Verification items for the finished model (mm, model axes). A direction names the side the tool comes from. Coordinates: 2 decimals unless noted, no trailing zeros. Loops run counter-clockwise (first coordinate to the right, second up) from the corner with the lowest first, then second, coordinate; pieces in that order, holes last. Notation, with made-up numbers: (32.25, 78.25) - (64.25, 78.25) arc R19 ccw to (64.25, 82.25) - close; hole circle Ø2 at (3.25, 41.5). An arc over 180 degrees is marked (long way). One line per item, written item: value. Start each with the question number.
(1) Draft check along Z on faces 3 (the face through (3.544, -43.056, 40.685)), 4 (the face through (16.244, -69.867, 15.456)), 5 (the face through (3.544, -77.418, 26.011)), 6 (the face through (-2.717, -36, 1)). Enter one of: +Z half, -Z half, draft (parallel to the pull), parting line (faces both ways), or undercut.
(2) Set-up check for faces 1 (the face through (9.983, -22, 1)), 2 (the face through (3.5, -14.1, 0.8)): record each of +Z, -Z, +X, -X, +Y, -Y from which the full face is reachable in a straight line by a thin tool's end or side.
(3) Thickness scan on probe 1 along Z at (x, y) = (7, -58.5); probe 2 along Z at (x, y) = (9.75, -68); probe 3 along Y at (x, z) = (15, 1). Record the ranges inside material, lowest first. Write a range as [from, to].
(4) Section check D-D (z = -56). Record the boundary of the cut face in (x, y), plus the area to 3 significant figures.
(5) Gauge pin test, flat ends, axial feed: P1, Ø10, axis at y = -15.8, z = 24.63, coming from the +X side; P2, Ø14.5, axis at y = -36.76, z = -39.86, coming from the +X side; P3, Ø16.5, axis at y = -91.62, z = 0, coming from the -X side; P4, Ø1, axis at x = 9.5, z = -43.5, coming from the -Y side. Record the tip position at first contact, or that the pin passes through.
(6) Section check B-B (x = 20.75). Record the boundary of the cut face in (y, z) (3 decimals), plus the area to 3 significant figures.
(7) Section check A-A (x = 1.75). Count the separate pieces of the cut face and the enclosed holes in it, plus the area to 3 significant figures.
(8) Section check C-C (z = 49.5). Record the boundary of the cut face in (x, y).
Autodesk Inventor part; units mm, degrees
ref_plane "YZ Plane" through (0, 0, 0) normal (1, 0, 0) x (0, 1, 0)
ref_plane "XZ Plane" through (0, 0, 0) normal (0, 1, 0) x (-1, 0, 0)
ref_plane "XY Plane" through (0, 0, 0) normal (0, 0, 1) x (1, 0, 0)
sketch "Sketch1" plane through (0, 0, 0) normal (0, 0, 1) x (1, 0, 0)
  line L0 (-2.7173, 13.7894) -> (9.9827, 13.7894)
  line L1 (9.9827, 13.7894) -> (9.9827, -24.3106)
  line L2 (9.9827, -40.1856) -> (-2.7173, -40.1856)
  line L3 (-2.7173, -40.1856) -> (-2.7173, 13.7894)
  line L4 (-2.7173, -40.1856) -> (22.6827, -40.1856)
  line L5 (22.6827, -40.1856) -> (22.6827, -24.3106)
  line L6 (22.6827, -24.3106) -> (9.9827, -24.3106)
  line L7 (-2.7173, -24.3106) -> (-2.7173, -40.1856)
  line L8 (-16.1487, -49.7106) -> (31.6829, -49.7106)
  point P0 (0, 0)
  dimension "d0" = 12.7
  dimension "d1" = 53.975
  dimension "d4" = 25.4
  dimension "d5" = 15.875
  dimension "d6" = 9.525
revolve "Revolution1" add sketch "Sketch1" angle 360 about axis through (-16.1487, -49.7106, 0) along (1, 0, 0)
sketch "Sketch3" plane through (22.6827, -49.7106, 0) normal (1, 0, 0) x (0, 0, -1)
  line L0 (0, 11.43) -> (-1.27, 11.43)
  line L1 (0, 11.43) -> (1.27, 11.43)
  line L2 (1.27, 11.43) -> (1.27, 9.44)
  circle A0 centre (0, 0) radius 9.525
  line L3 (-1.27, 11.43) -> (-1.27, 9.44)
  line L4 (1.27, 9.44) -> (-1.27, 9.44)
  point P0 (0, 49.7106)
  dimension "d9" = 1.27
  dimension "d10" = 1.27
extrude "Extrusion1" cut sketch "Sketch3" against normal blind 25.4 contours L1 L2 A0 L3 L0
sketch "Sketch7" plane through (22.6827, -49.7106, 0) normal (1, 0, 0) x (0, 0, -1)
  point P0 (0, 49.7106)
  point P1 (0, 0)
  point P2 (0, 41.91)
  point P3 (-24.6341, 33.9059)
  point P4 (-39.8588, 12.9509)
  point P5 (-39.8588, -12.9509)
  point P6 (-24.6341, -33.9059)
  point P7 (0, -41.91)
  point P8 (24.6341, -33.9059)
  point P9 (39.8588, -12.9509)
  point P10 (39.8588, 12.9509)
  point P11 (24.6341, 33.9059)
  dimension "d29" = 41.91
  dimension "d32" = 360
hole "Hole3" at (22.6827, -49.7106, 0) at (22.6827, -7.8006, 0) at (22.6827, -15.8047, 24.6341) at (22.6827, -36.7597, 39.8588) at (22.6827, -62.6615, 39.8588) at (22.6827, -83.6165, 24.6341) at (22.6827, -91.6206, 0) at (22.6827, -83.6165, -24.6341) at (22.6827, -62.6615, -39.8588) at (22.6827, -36.7597, -39.8588) at (22.6827, -15.8047, -24.6341) direction (-1, 0, 0) diameter 12.7 end through all
properties part number "arthurWeiActivity 5.5a#4.dwg"
Responses:
1. face 3: undercut
1. face 4: parting line
1. face 5: undercut
1. face 6: draft
2. face 1: +X
2. face 2: +X, -X
3. probe 1: z = [-62.89, -44.66], [-35.06, -3.67], [3.67, 35.06], [44.66, 62.89]
3. probe 2: z = [-60.81, -43.3], [-36.42, 36.42], [43.3, 60.81]
3. probe 3: y = [-75.09, -59.18], [-38.28, -24.33]
4. outline: (-2.72, -79.65) - (9.98, -79.65) - (9.98, -19.77) - (-2.72, -19.77) - close
4. area: 760 mm²
5. P1: passes through
5. P2: stops at x = 9.98
5. P3: stops at x = -2.72
5. P4: stops at y = -96.44
6. outline: circle Ø50.8 at (-49.711, 0); hole (-40.271, -1.27) - (-38.281, -1.27) - (-38.281, 1.27) - (-40.271, 1.27) arc R9.525 ccw (long way) to start
6. area: 1,740 mm²
7. separate pieces: 1
7. enclosed holes: 11
7. area: 11,100 mm²
8. outline: (-2.72, -89.48) - (9.98, -89.48) - (9.98, -9.94) - (-2.72, -9.94) - close
